The model under review builds one solid part; all positions refer to its coordinate system, in mm. A direction names the side the tool comes from. Coordinates: 2 decimals unless noted, no trailing zeros. Order: outer loops, then holes, each group sorted by start corner. A loop starts at its lowest first (then second) coordinate and runs counter-clockwise, first axis right, second up.
```python
from build123d import *

# Parameters (mm, degrees)
F0_W     = 44.45
F0_H     = 16.51
F0_R     = 2.2225
F1_DEPTH = 3.81
F2_W     = 44.45
F2_H     = 12.7
F2_R     = 2.2225
F3_DEPTH = 3.81
F4_SIZE  = 1.27
F5_SIZE  = 1.27


with BuildPart() as f1:
    # F0 (on Top) → F1 (new body)
    with BuildSketch(Plane.XY):
        with Locations((22.225, 8.255)):
            Rectangle(F0_W, F0_H)
        with Locations((16.9164, 10.16)):
            Circle(F0_R, mode=Mode.SUBTRACT)
        with Locations((38.1, 10.16)):
            Circle(F0_R, mode=Mode.SUBTRACT)
    extrude(amount=F1_DEPTH)

    # F2 (on face) → F3 (join)
    with BuildSketch(Plane.XZ):
        with Locations((22.225, 10.16)):
            Rectangle(F2_W, F2_H)
        with Locations((6.35, 10.16)):
            Circle(F2_R, mode=Mode.SUBTRACT)
        with Locations((27.5336, 10.16)):
            Circle(F2_R, mode=Mode.SUBTRACT)
    extrude(amount=-F3_DEPTH)

    # F4
    f4_edges = [f1.edges().sort_by_distance(p)[0] for p in [
        (22.225, 0, 0),
    ]]
    chamfer(f4_edges, length=F4_SIZE)

    # F5
    f5_edges = [f1.edges().sort_by_distance(p)[0] for p in [
        (22.225, 3.81, 3.81),
    ]]
    chamfer(f5_edges, length=F5_SIZE)


solid = f1.part
```
(1) We need section C-C, the plane y = 2. Count the separate pieces of the cut face and the enclosed holes in it, and give its area (3 significant figures).
A:
separate pieces: 1
enclosed holes: 2
area: 703 mm2
(2) Draft analysis for pull direction X (two halves, no side actions). For faces 1 (the face through (44.45, 4, 3)), 2 (the face through (29.653, 1.878, 10.828)), 3 (the face through (6.061, 1.878, 12.364)), 4 (the face through (22, 16.51, 2)), state which applies: released by +X, released by -X, zero draft, split by the parting line, or undercut.
A:
face 1: released by +X
face 2: undercut
face 3: undercut
face 4: zero draft
(3) For pin 1 Ø9 at (x, z) = (21, 11.5) entering from +Y; pin 2 Ø4 at (x, y) = (38.1, 10.16) entering from -Z; pin 3 Ø5 at (x, y) = (16.92, 10.16) entering from +Z; pin 4 Ø9 at (x, y) = (33, 9.5) entering from +Z, all flat-tipped, find the tip position at first contact; note any pin that passes through.
A:
pin 1: stops at y = 3.81
pin 2: passes through
pin 3: stops at z = 3.81
pin 4: stops at z = 3.89
(4) We need section B-B, the plane x = 38.1. Write out the cut boundary in (y, z).
A:
outline: (0, 1.27) - (1.27, 0) - (7.94, 0) - (7.94, 3.81) - (5.08, 3.81) - (3.81, 5.08) - (3.81, 16.51) - (0, 16.51) - close; (12.38, 0) - (16.51, 0) - (16.51, 3.81) - (12.38, 3.81) - close
(5) We need section D-D, the plane y = 11. Write out the cut boundary in (x, z).
A:
outline: (0, 0) - (14.86, 0) - (14.86, 3.81) - (0, 3.81) - close; (18.97, 0) - (36.04, 0) - (36.04, 3.81) - (18.97, 3.81) - close; (40.16, 0) - (44.45, 0) - (44.45, 3.81) - (40.16, 3.81) - close
(6) Machinability: for faces 5 (the face through (22, 9, 0)), 6 (the face through (22, 3.81, 11)), which of the approach directions +Z, -Z, +X, -X, +Y, -Y give a long, thin tool a straight path to every point of the face, cutting with its end or side? Answer none if there is none.
A:
face 5: -Z, +X, -X, +Y, -Y
face 6: +Z, +X, -X, +Y
(7) Wall thickness on probe 1 along Y at (x, z) = (38, 2.5); probe 2 along Z at (x, y) = (39, 7.75): over which ranges is each line inside the solid? List them lowest first.
A:
probe 1: y = 0 to 7.94, 12.38 to 16.51
probe 2: z = 0 to 3.81
(8) We need section A-A, the plane z = 10.16. Write out the cut boundary in (x, y).
A:
outline: (0, 0) - (4.13, 0) - (4.13, 3.81) - (0, 3.81) - close; (8.57, 0) - (25.31, 0) - (25.31, 3.81) - (8.57, 3.81) - close; (29.76, 0) - (44.45, 0) - (44.45, 3.81) - (29.76, 3.81) - close
